```python
from build123d import *

# Parameters (mm, degrees)
SKETCH3_R          = 2
CUT_EXTRUDE1_DEPTH = 32
CIRPATTERN1_COUNT  = 8
CHAMFER1_SIZE      = 0.5
CHAMFER2_SIZE      = 0.5


with BuildPart() as part:
    # Sketch2 → Revolve1 (revolve)
    with BuildSketch(Plane(origin=(0, 0, 0), x_dir=(1, 0, 0), z_dir=(0, 1, 0)), mode=Mode.PRIVATE) as revolve1_sk:
        Polygon((0, 30), (0, 48), (-32, 48), (-32, 37.5), (-44.5, 37.5), (-44.5, 0), (-42.5, 0), (-42.5, 11), (-36.5, 11), (-36.5, 8), (-8, 8), (-8, 21), (2, 21), (2, 30), align=None)
    revolve(revolve1_sk.sketch.rotate(Axis((-32, 0, 0), (1, 0, 0)), 180), axis=Axis((-32, 0, 0), (1, 0, 0)))

    # Sketch3 → Cut-Extrude1 (cut)
    with BuildSketch(Plane.ZY.offset(32)):
        with Locations((0, 42)):
            Circle(SKETCH3_R)
    cut_extrude1 = extrude(amount=-CUT_EXTRUDE1_DEPTH, mode=Mode.SUBTRACT)

    # CirPattern1: Cut-Extrude1 ×8 about axis
    cirpattern1_axis = Axis((0, 0, 0), (1, 0, 0))
    for i in range(1, CIRPATTERN1_COUNT):
        add(cut_extrude1.rotate(cirpattern1_axis, i * 360 / CIRPATTERN1_COUNT), mode=Mode.SUBTRACT)

    # Chamfer1
    chamfer1_edges = [part.edges().sort_by_distance(p)[0] for p in [
        (-44.5, 0, -37.5),
        (-32, 0, -48),
        (0, 0, -48),
    ]]
    chamfer(chamfer1_edges, length=CHAMFER1_SIZE)

    # Chamfer2
    chamfer2_edges = [part.edges().sort_by_distance(p)[0] for p in [
        (2, 0, -30),
    ]]
    chamfer(chamfer2_edges, length=CHAMFER2_SIZE)


solid = part.part
```
Verification items for the finished model (mm, model axes). A direction names the side the tool comes from. Round coordinates to 2 decimals unless told otherwise and drop trailing zeros. Order: outer loops, then holes, each group sorted by start corner. A loop starts at its lowest first (then second) coordinate and runs counter-clockwise, first axis right, second up. Notation, with made-up numbers: (24, 54) -> (32, 54) arc R13 ccw to (32, 74) -> close; hole circle Ø8 at (-3.5, 79.5). An arc over 180 degrees is marked (long way). Put each result on its own line as item: value. Start each with the question number.
(1) Draft check along Z on faces 1 (the face through (-44.5, -1, -1)), 2 (the face through (-39.46, 10.74, -2.38)), 3 (the face through (-16.217, -14.418, 45.783)). Enter one of: +Z half, -Z half, draft (parallel to the pull), parting line (faces both ways), or undercut.
(2) Material ranges on line 1 along Y through (x, z) = (-26, -1.5); line 2 along X through (y, z) = (-33, 28); line 3 along Z through (x, y) = (-16, 29), recorded low to high.
(3) Tool access check on faces 4 (the face through (-22.05, 7.81, -1.73)), 5 (the face through (-36.5, 8, -2)), 6 (the face through (-16.224, 29.96, 27.716)). Record the directions out of +Z, -Z, +X, -X, +Y, -Y that give a thin tool (end or side, any length) a straight path to the whole face; none if there is none.
(4) Section check A-A (z = 0). State how many separate pieces and enclosed holes the cut face has, then the cut area to 3 significant figures.
(5) Depth check by flat-ended pin: pin 1 Ø5 at (x, y) = (-13.5, 25) entering from +Z; pin 2 Ø5 at (y, z) = (42, 0) entering from -X; pin 3 Ø4 at (x, z) = (-16, 29) entering from +Y; pin 4 Ø2.5 at (y, z) = (29.7, 29.7) entering from +X. Enter the tip coordinate at first touch or a pass-through.
(6) Section check D-D (x = -35). Enter the section's corners in (y, z).
Completed:
1. face 1: draft
1. face 2: undercut
1. face 3: parting line
2. line 1: y = -47.98 to -43.32, -40.68 to -7.86, 7.86 to 40.68, 43.32 to 47.98
2. line 2: x = -32 to 0
2. line 3: z = -38.25 to -31.57, -27.82 to 27.82, 31.57 to 38.25
3. face 4: +X
3. face 5: none
3. face 6: +X, -X
4. separate pieces: 3
4. enclosed holes: 0
4. area: 2,860 mm2
5. pin 1: stops at z = 42.4
5. pin 2: stops at x = -32
5. pin 3: stops at y = 39.69
5. pin 4: passes through
6. outline: circle Ø75 at (0, 0); hole circle Ø16 at (0, 0)
